Geometry check sheet. Reference: the model listing, model coordinates, mm. Round coordinates to 2 decimals unless told otherwise and drop trailing zeros. Write each loop counter-clockwise with the first axis right and the second up, starting at its lowest first coordinate (ties: lowest second). Pieces come first, ordered by that corner, then holes. Notation, with made-up numbers: M -32,25.25 L -18,25.25 A26 ccw -18,43.25 Z; hole C 24,72.25 d1. An arc over 180 degrees is marked long. Answer in a Markdown table with one row per item. Add a question column.
from build123d import *

# Parameters (mm, degrees)
SKETCH1_R           = 6
BOSS_EXTRUDE1_DEPTH = 63.5
SKETCH3_W           = 1.4
SKETCH3_H           = 2.2
CUT_EXTRUDE1_DEPTH  = 50.8
FILLET1_R           = 6.35


with BuildPart() as part:
    # Sketch1 → Boss-Extrude1 (new body)
    with BuildSketch(Plane.XY):
        Circle(SKETCH1_R)
    extrude(amount=BOSS_EXTRUDE1_DEPTH)

    # Sketch2 → Revolve1 (revolve)
    with BuildSketch(Plane(origin=(0, 0, 0), x_dir=(0, 0, -1), z_dir=(1, 0, 0))):
        with BuildLine():
            Line((-63.5, 0), (-113.581166909, 0))
            ThreePointArc((-113.581166909, 0), (-91.202620244, 25.21965146), (-63.5, 6))
            Line((-63.5, 6), (-63.5, 0))
        make_face()
    revolve(axis=Axis((0, 0, 63.5), (0, 0, 1)))

    # Sketch3 → Cut-Extrude1 (cut)
    with BuildSketch(Plane(origin=(0, 0, 0), x_dir=(-1, 0, 0), z_dir=(0, 0, -1))):
        Rectangle(SKETCH3_W, SKETCH3_H)
    extrude(amount=-CUT_EXTRUDE1_DEPTH, mode=Mode.SUBTRACT)

    # Fillet1
    fillet1_edges = [part.edges().sort_by_distance(p)[0] for p in [
        (-4.242640687, -4.242640687, 63.5),
    ]]
    fillet(fillet1_edges, radius=FILLET1_R)


solid = part.part
Item 1: Gauge pin test, flat ends, axial feed: pin 1 Ø10 at (y, z) = (11, 66.5) entering from +X; pin 2 Ø2 at (x, y) = (-11, -13.5) entering from +Z; pin 3 Ø10 at (x, y) = (1, -9.5) entering from +Z. Record the tip position at first contact, or that the pin passes through.
Item 2: Section check A-A, the plane z = 106. Record the boundary of the cut face in (x, y).
Item 3: Scan lines: probe 1 along X at (y, z) = (0.5, 47); probe 2 along Y at (x, z) = (0, 28.5); probe 3 along Y at (x, z) = (3, 31). Record each from-to range of solid material in increasing order. Write a range as from..to.
Item 4: Mould release check, pull along Y, two halves, no side actions. Record for faces 1 (the cylindrical face through (5.723, 1.802, 29.053)), 2 (the flat face through (1, 0, 0)), 3 (the flat face through (0.7, 0, 25)): +Y half, -Y half, draft (parallel to the pull), parting line (faces both ways), or undercut.
Item 5: Section check B-B, the plane x = -21.5. Record the boundary of the cut face in (y, z), and give its area (3 significant figures).
Result sheet:
| question | item | result |
|---|---|---|
| 1 | pin 1 | stops at x = 16.5 |
| 1 | pin 2 | stops at z = 107.57 |
| 1 | pin 3 | stops at z = 113.17 |
| 2 | outline | C 0,0 d36.2 |
| 3 | probe 1 | x = -5.98..-0.7, 0.7..5.98 |
| 3 | probe 2 | y = -6..-1.1, 1.1..6 |
| 3 | probe 3 | y = -5.2..5.2 |
| 4 | face 1 | parting line |
| 4 | face 2 | draft |
| 4 | face 3 | undercut |
| 5 | outline | C 0,88.18 d27.05 |
| 5 | area | 575 mm^2 |
